Check sheet for the modelled part. Datum: model origin and axes. Units: mm. Coordinates: 2 decimals unless noted, no trailing zeros. Write each loop counter-clockwise with the first axis right and the second up, starting at its lowest first coordinate (ties: lowest second). Pieces come first, ordered by that corner, then holes. Notation, with made-up numbers: M 54.5,-40 L 92.5,-40 A20 cw 92.5,-31 Z; hole C 80,5.5 d7. An arc over 180 degrees is marked long. Answer as CSV lines item,"result".
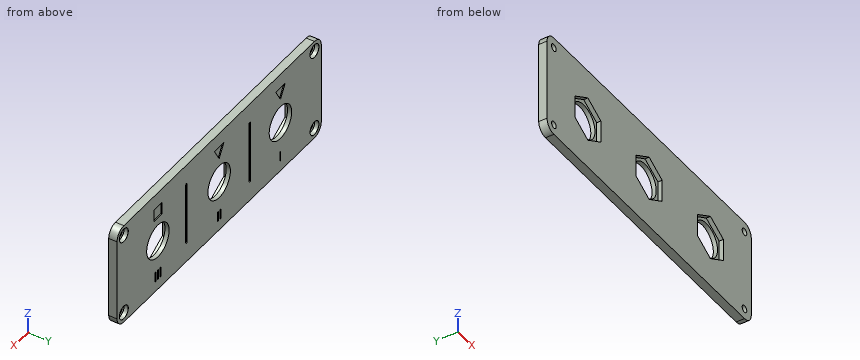
from build123d import *

# Parameters (mm, degrees)
SKETCH1_W                = 150
SKETCH1_H                = 50
BODY_DEPTH               = 4
EDGE_FILLETS_R           = 5
GX16_HOLE_D              = 16.5
GX16_NUT_CUTOUT_DEPTH    = 2
GX16_PATTERN_COUNT       = 3
GX16_PATTERN_PITCH       = 45
DESIGN_CUTOUT_SKETCH_W   = 6
DESIGN_CUTOUT_SKETCH_H   = 6
DESIGN_CUTOUT_SKETCH_W_2 = 0.641025641
DESIGN_CUTOUT_SKETCH_H_2 = 5
DESIGN_CUTOUT_DEPTH      = 0.5


# Read off the part's stored shape, not the designer's step: mounting_holes
with BuildPart() as part:
    # Sketch1 → body (new body)
    with BuildSketch(Plane(origin=(0, 0, 0), x_dir=(1, 0, 0), z_dir=(0, 1, 0))):
        Rectangle(SKETCH1_W, SKETCH1_H)
    extrude(amount=BODY_DEPTH)

    # mounting_holes outline → mounting_holes (revolve, cut)
    with BuildSketch(Plane(origin=(70, 0, 20), x_dir=(1, 0, 0), z_dir=(0, 0, 1))):
        Polygon((0, 0), (1.7, 0), (1.7, 2), (3.25, 2), (3.25, 3.975), (3.275, 4), (0, 4), align=None)
    revolve(axis=Axis((70, 0, 20), (0, 1, 0)), mode=Mode.SUBTRACT)

    # mounting_holes 2 outline → mounting_holes 2 (revolve, cut)
    with BuildSketch(Plane(origin=(-70, 0, -20), x_dir=(1, 0, 0), z_dir=(0, 0, 1))):
        Polygon((0, 4), (0, 0), (1.7, 0), (1.7, 2), (3.25, 2), (3.25, 3.975), (3.275, 4), align=None)
    revolve(axis=Axis((-70, 0, -20), (0, 1, 0)), mode=Mode.SUBTRACT)

    # mounting_holes 3 outline → mounting_holes 3 (revolve, cut)
    with BuildSketch(Plane(origin=(70, 0, -20), x_dir=(1, 0, 0), z_dir=(0, 0, 1))):
        Polygon((0, 4), (0, 0), (1.7, 0), (1.7, 2), (3.25, 2), (3.25, 3.975), (3.275, 4), align=None)
    revolve(axis=Axis((70, 0, -20), (0, 1, 0)), mode=Mode.SUBTRACT)

    # mounting_holes 4 outline → mounting_holes 4 (revolve, cut)
    with BuildSketch(Plane(origin=(-70, 0, 20), x_dir=(1, 0, 0), z_dir=(0, 0, 1))):
        Polygon((0, 4), (0, 0), (1.7, 0), (1.7, 2), (3.25, 2), (3.25, 3.975), (3.275, 4), align=None)
    revolve(axis=Axis((-70, 0, 20), (0, 1, 0)), mode=Mode.SUBTRACT)

    # edge_fillets
    edge_fillets_edges = [part.edges().sort_by_distance(p)[0] for p in [
        (75, 2, 25),
        (-75, 2, 25),
        (-75, 2, -25),
        (75, 2, -25),
    ]]
    fillet(edge_fillets_edges, radius=EDGE_FILLETS_R)

    # gx16_hole (through all)
    with Locations(Plane(origin=(0, 4, 0), x_dir=(1, 0, 0), z_dir=(0, 1, 0))):
        with Locations((-45, 0)):
            gx16_hole = Hole(GX16_HOLE_D / 2)

    # Sketch6 → gx16_nut-cutout (cut)
    with BuildSketch(Plane.XZ):
        Polygon((-45, 10.969655115), (-54.5, 5.484827557), (-54.5, -5.484827557), (-45, -10.969655115), (-35.5, -5.484827557), (-35.5, 5.484827557), align=None)
    gx16_nut_cutout = extrude(amount=-GX16_NUT_CUTOUT_DEPTH, mode=Mode.SUBTRACT)

    # gx16_pattern: gx16_hole, gx16_nut-cutout ×3
    with Locations(*[(i * GX16_PATTERN_PITCH, 0, 0) for i in range(1, GX16_PATTERN_COUNT)]):
        add(gx16_hole, mode=Mode.SUBTRACT)
        add(gx16_nut_cutout, mode=Mode.SUBTRACT)

    # design_cutout_sketch → design_cutout (cut)
    with BuildSketch(Plane(origin=(0, 4, 0), x_dir=(1, 0, 0), z_dir=(0, 1, 0))):
        with BuildLine():
            Line((-22, 15), (-22, -15))
            ThreePointArc((-22, -15), (-22.5, -15.5), (-23, -15))
            Line((-23, -15), (-23, 15))
            ThreePointArc((-23, 15), (-22.5, 15.5), (-22, 15))
        make_face()
        with BuildLine():
            Line((24.543317326, 15), (24.543317326, -15))
            ThreePointArc((24.543317326, -15), (24.043317326, -15.5), (23.543317326, -15))
            Line((23.543317326, -15), (23.543317326, 15))
            ThreePointArc((23.543317326, 15), (24.043317326, 15.5), (24.543317326, 15))
        make_face()
        with Locations((45, -15)):
            Rectangle(DESIGN_CUTOUT_SKETCH_W, DESIGN_CUTOUT_SKETCH_H)
        Polygon((0, -12), (-3.464101615, -18), (3.464101615, -18), align=None)
        Polygon((-45, -12), (-48.464101615, -18), (-41.535898385, -18), align=None)
        with Locations((-44.903846154, 17.5)):
            Rectangle(DESIGN_CUTOUT_SKETCH_W_2, DESIGN_CUTOUT_SKETCH_H_2)
        with Locations((-0.969230769, 17.5)):
            Rectangle(DESIGN_CUTOUT_SKETCH_W_2, DESIGN_CUTOUT_SKETCH_H_2)
        with Locations((0.825641025, 17.5)):
            Rectangle(DESIGN_CUTOUT_SKETCH_W_2, DESIGN_CUTOUT_SKETCH_H_2)
        with Locations((43.211538462, 17.5)):
            Rectangle(DESIGN_CUTOUT_SKETCH_W_2, DESIGN_CUTOUT_SKETCH_H_2)
        with Locations((45.006410257, 17.5)):
            Rectangle(DESIGN_CUTOUT_SKETCH_W_2, DESIGN_CUTOUT_SKETCH_H_2)
        with Locations((46.801282052, 17.5)):
            Rectangle(DESIGN_CUTOUT_SKETCH_W_2, DESIGN_CUTOUT_SKETCH_H_2)
    extrude(amount=-DESIGN_CUTOUT_DEPTH, mode=Mode.SUBTRACT)


solid = part.part
1) Section check C-C, the plane z = -3. Give the number of separate pieces and of enclosed holes in the cut face, plus the area to 3 significant figures.
Answer key:
separate pieces,"4"
enclosed holes,"0"
area,"393 mm2"
2) Thickness scan on line 1 along Z through (x, y) = (-70, 1.35); line 2 along X through (y, z) = (1.3, -5.5); line 3 along Z through (x, y) = (-45, 2.85). Record the ranges inside material, lowest first.
Answer key:
line 1,"z = -25 to -21.7, -18.3 to 18.3, 21.7 to 25"
line 2,"x = -75 to -54.47, -35.53 to -9.47, 9.47 to 35.53, 54.47 to 75"
line 3,"z = -25 to -8.25, 8.25 to 25"
3) Section check A-A, the plane x = 50. Record the boundary of the cut face in (y, z).
Answer key:
outline,"M 0,-25 L 4,-25 L 4,-6.56 L 2,-6.56 L 2,-8.08 L 0,-8.08 Z; M 0,8.08 L 2,8.08 L 2,6.56 L 4,6.56 L 4,25 L 0,25 Z"
4) Depth check by flat-ended pin: P1, Ø5.5, axis at x = 70, z = -20, coming from the -Y side. Enter the tip coordinate at first touch or a pass-through.
Answer key:
P1,"stops at y = 0"
5) Section check B-B, the plane y = 2.9. Record the boundary of the cut face in (x, z).
Answer key:
outline,"M -75,-20 A5 ccw -70,-25 L 70,-25 A5 ccw 75,-20 L 75,20 A5 ccw 70,25 L -70,25 A5 ccw -75,20 Z; hole C -70,-20 d6.5; hole C -70,20 d6.5; hole C -45,0 d16.5; hole C 0,0 d16.5; hole C 45,0 d16.5; hole C 70,-20 d6.5; hole C 70,20 d6.5"
